Build history of the part. All positions in model axes, mm. A direction names the side the tool comes from. Give positions to 0.01 mm unless a question says otherwise; leave off trailing zeros. Loops run counter-clockwise (first coordinate to the right, second up) from the corner with the lowest first, then second, coordinate; pieces in that order, holes last. Notation, with made-up numbers: M 41,33.5 L 61,33.5 A25 ccw 61,58.5 Z; hole C 41.25,57 d2. An arc over 180 degrees is marked long. Answer as a JSON object with one key per item and string values. Group by question number.
1. Slice it at B-B (z = 440). List the corners of the cut face in (x, y), then the cut area to 3 significant figures.
2. Slice it at A-A (x = -1). List the corners of the cut face in (y, z), then the cut area to 3 significant figures.
3. 3-axis set-ups, long thin cutter, end or side, ignore diameter. For faces 5 (the face through (-0.1, 8.2, 0)), 6 (the face through (0, -8, 659)): which of +Z, -Z, +X, -X, +Y, -Y reach the whole face in a straight line?
4. Drill centre lines: line 1 along X through (y, z) = (-8.65, 10); line 2 along Y through (x, z) = (-16, 787); line 3 along X through (y, z) = (-6.75, 1090.5). Where is each one in solid material? Low to high. Write a range as [from, to].
5. Mould opens along X. For faces 1 (the face through (-25, 0, 641)), 2 (the face through (0, 8, 659)), 3 (the face through (25, 0, 641)), 4 (the face through (0, -10, 641)) say: released by +X, released by -X, zero draft, split by the parting line, or undercut.
6. Slice it at C-C (y = 4.25). List the corners of the cut face in (x, z), then the cut area to 3 significant figures.
from build123d import *

# Parameters (mm, degrees)
SKETCH_1_W          = 50
SKETCH_1_H          = 20
EXTRUDE_1_DEPTH     = 1300
SKETCH_2_W          = 46
SKETCH_2_H          = 16
CUT_EXTRUDE_1_DEPTH = 1301.278816254
SKETCH_3_R          = 4.80233269
SKETCH_3_R_2        = 4.787191165
SKETCH_3_R_3        = 5.290306375
SKETCH_3_R_4        = 4.870795403
CUT_EXTRUDE_2_DEPTH = 1301.394171011


with BuildPart() as part:
    # Sketch 1 → Extrude 1 (new body)
    with BuildSketch(Plane.XY):
        Rectangle(SKETCH_1_W, SKETCH_1_H)
    extrude(amount=EXTRUDE_1_DEPTH)

    # Sketch 2 → Cut-Extrude 1 (cut, through all)
    with BuildSketch(Plane.XY.offset(1300)):
        Rectangle(SKETCH_2_W, SKETCH_2_H)
    extrude(amount=-CUT_EXTRUDE_1_DEPTH, mode=Mode.SUBTRACT)

    # Sketch 3 → Cut-Extrude 2 (cut, through all)
    with BuildSketch(Plane(origin=(0, 10, 0), x_dir=(1, 0, 0), z_dir=(0, 1, 0))):
        with Locations(Location((15, -1290, 0), (0, 0, 270))):
            Circle(SKETCH_3_R)
        with Locations(Location((-15, -1290, 0), (0, 0, 270))):
            Circle(SKETCH_3_R_2)
        with Locations(Location((15, -1260, 0), (0, 0, 270))):
            Circle(SKETCH_3_R_3)
        with Locations(Location((-15, -1260, 0), (0, 0, 270))):
            Circle(SKETCH_3_R_4)
        with Locations(Location((15, -10, 0), (0, 0, 270))):
            Circle(SKETCH_3_R_4)
        with Locations(Location((-15, -10, 0), (0, 0, 270))):
            Circle(SKETCH_3_R_4)
        with Locations(Location((15, -40, 0), (0, 0, 270))):
            Circle(SKETCH_3_R_4)
        with Locations(Location((-15, -40, 0), (0, 0, 270))):
            Circle(SKETCH_3_R_4)
    extrude(amount=-CUT_EXTRUDE_2_DEPTH, mode=Mode.SUBTRACT)


solid = part.part
Established:
{
 "1": {"outline": "M -25,-10 L 25,-10 L 25,10 L -25,10 Z; hole M -23,-8 L 23,-8 L 23,8 L -23,8 Z", "area": "264 mm^2"},
 "2": {"outline": "M -10,0 L -8,0 L -8,1300 L -10,1300 Z; M 8,0 L 10,0 L 10,1300 L 8,1300 Z", "area": "5,200 mm^2"},
 "3": {"face 5": "-Z, +X, -X, +Y, -Y", "face 6": "+Z, -Z"},
 "4": {"line 1": "x = [-25, -19.87], [-10.13, 10.13], [19.87, 25]", "line 2": "y = [-10, -8], [8, 10]", "line 3": "x = [-25, -23], [23, 25]"},
 "5": {"face 1": "released by -X", "face 2": "undercut", "face 3": "released by +X", "face 4": "zero draft"},
 "6": {"outline": "M -25,0 L -23,0 L -23,1300 L -25,1300 Z; M 23,0 L 25,0 L 25,1300 L 23,1300 Z", "area": "5,200 mm^2"}
}
